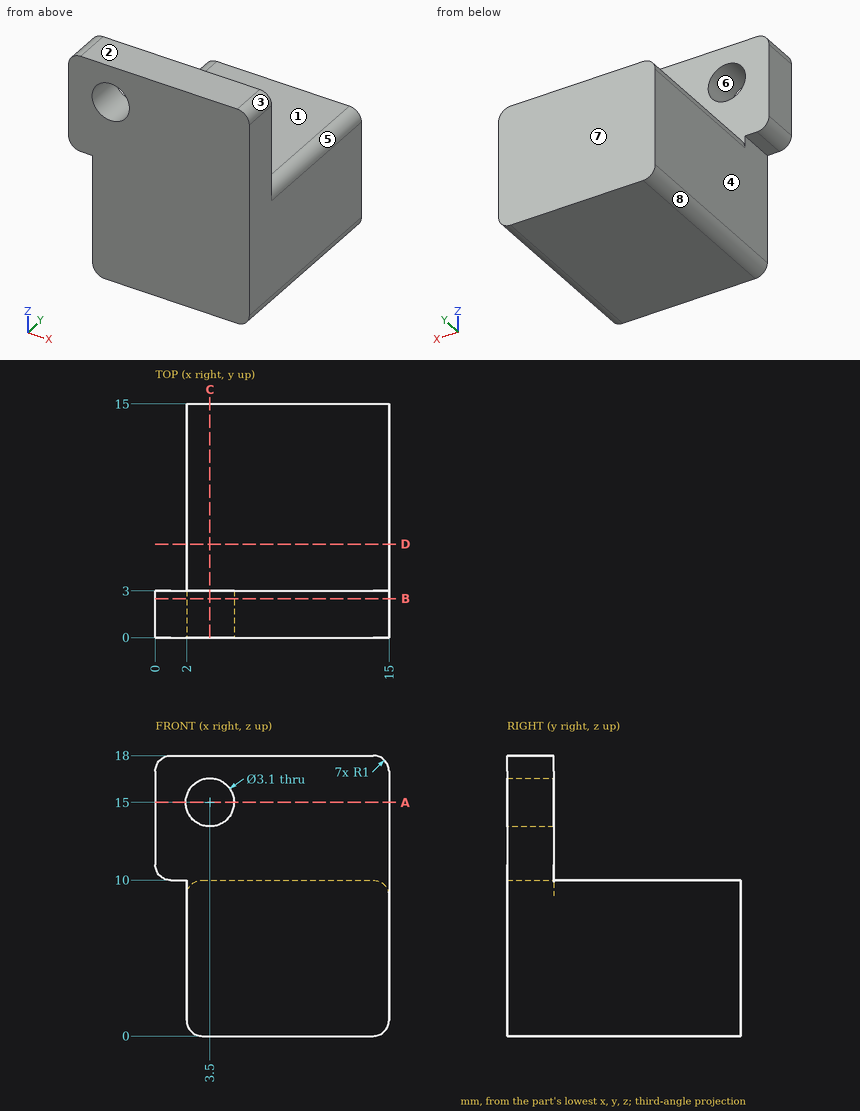
Geometry: see drawing. Coordinates: mm, zero at the bounding-box minimum. A direction names the side the tool comes from. Round coordinates to 2 decimals unless told otherwise and drop trailing zeros. Write each loop counter-clockwise with the first axis right and the second up, starting at its lowest first coordinate (ties: lowest second). Pieces come first, ordered by that corner, then holes. Notation, with made-up numbers: M -4,-28 L 20,-28 A16 cw 20,-14 Z; hole C 78,30 d11. An arc over 180 degrees is marked long. Answer as a JSON object with one key per item and string values. Group by question number.
(1) Section query C-C on x = 3.5. Output: boundary loops of the cut face in (y, z).
(2) First-contact query: pin 1 (1 mm diameter, centred on y = 8.5, z = 10, fed in from -X); pin 2 (2.5 mm diameter, centred on y = 4, z = 6, fed in from -X); pin 3 (2.5 mm diameter, centred on x = 8.5, z = 14.5, fed in from +Y). Flat tips, straight axial feed; report the tip coordinate or a pass-through.
(3) Reachability of the marked faces 1, 2, 3, 4 and 5 from +Z, -Z, +X, -X, +Y, -Y: full face, straight path, thin tool, end or side. Return the list, or none.
(4) Ray query, line 1 (X direction, y = 2.2, z = 15); line 2 (Y direction, x = 13.5, z = 13.75); line 3 (Z direction, x = 8.75, y = 6). Return the intervals inside material, ascending. Write a range as [from, to].
(5) Mould query, pull axis Z, two halves, no side actions, for the marked faces 6, 7 and 8. Classes: +Z half, -Z half, draft (parallel to the pull), parting line (faces both ways), or undercut.
(6) Section query A-A on z = 15. Output: boundary loops of the cut face in (x, y), then the cut area to 3 significant figures.
(7) Section query B-B on y = 2.5. Output: boundary loops of the cut face in (x, z), then the cut area to 3 significant figures.
(8) Section query D-D on y = 6. Output: boundary loops of the cut face in (x, z), then the cut area to 3 significant figures.
Computed values:
{
 "1": {"outline": "M 0,0 L 15,0 L 15,10 L 3,10 L 3,13.45 L 0,13.45 Z; M 0,16.55 L 3,16.55 L 3,18 L 0,18 Z"},
 "2": {"pin 1": "x = 2.13", "pin 2": "x = 2", "pin 3": "y = 3"},
 "3": {"face 1": "+Z, +X, -X, +Y", "face 2": "+Z, +X, -X, +Y, -Y", "face 3": "+Z, +X, +Y, -Y", "face 4": "-Z, -X, +Y, -Y", "face 5": "+Z, +X, +Y"},
 "4": {"line 1": "[0, 1.95], [5.05, 15]", "line 2": "[0, 3]", "line 3": "[0, 10]"},
 "5": {"face 6": "undercut", "face 7": "draft", "face 8": "-Z half"},
 "6": {"outline": "M 0,0 L 1.95,0 L 1.95,3 L 0,3 Z; M 5.05,0 L 15,0 L 15,3 L 5.05,3 Z", "area": "35.7 mm^2"},
 "7": {"outline": "M 0,11 A1 ccw 1,10 L 2,10 L 2,1 A1 ccw 3,0 L 14,0 A1 ccw 15,1 L 15,17 A1 ccw 14,18 L 1,18 A1 ccw 0,17 Z; hole C 3.5,15 d3.1", "area": "241 mm^2"},
 "8": {"outline": "M 2,1 A1 ccw 3,0 L 14,0 A1 ccw 15,1 L 15,9 A1 ccw 14,10 L 3,10 A1 ccw 2,9 Z", "area": "129 mm^2"}
}
